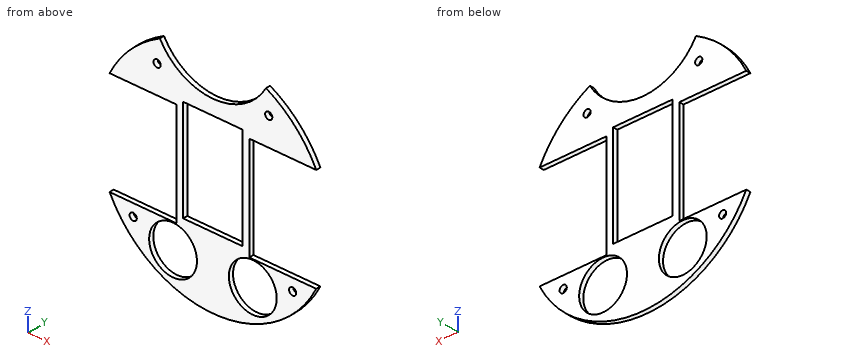
```python
from build123d import *

# Parameters (mm, degrees)
BOSS_EXTRUDE1_DEPTH  = 2.9
SOLENOID_PLACEMENT_W = 37.4
SOLENOID_PLACEMENT_H = 63.8
CUT_EXTRUDE1_DEPTH   = 103.571487266
CUT_EXTRUDE3_DEPTH   = 103.571487266
SKETCH7_R            = 15
CUT_EXTRUDE6_DEPTH   = 98.286484159
SKETCH8_R            = 2.25
CUT_EXTRUDE7_DEPTH   = 98.286484159


with BuildPart() as part:
    # Sketch1 → Boss-Extrude1 (new body)
    with BuildSketch(Plane(origin=(0, 0, 0), x_dir=(1, 0, 0), z_dir=(0, 1, 0))):
        with BuildLine():
            ThreePointArc((33.29110537, -64.404598464), (0, 72.5), (-33.29110537, -64.404598464))
            ThreePointArc((-33.29110537, -64.404598464), (0, -44.989799638), (33.29110537, -64.404598464))
        make_face()
    extrude(amount=BOSS_EXTRUDE1_DEPTH)

    # solenoid placement → Cut-Extrude1 (cut, through all)
    with BuildSketch(Plane(origin=(0, 2.9, 0), x_dir=(1, 0, 0), z_dir=(0, 1, 0))):
        with Locations((0, -3.8)):
            Rectangle(SOLENOID_PLACEMENT_W, SOLENOID_PLACEMENT_H)
    extrude(amount=-CUT_EXTRUDE1_DEPTH, mode=Mode.SUBTRACT)

    # Sketch3 → Cut-Extrude3 (cut, through all)
    with BuildSketch(Plane(origin=(0, 2.9, 0), x_dir=(1, 0, 0), z_dir=(0, 1, 0))):
        with BuildLine():
            Line((-34.63, -32.5), (-22.83, -32.5))
            Line((-22.83, -32.5), (-22.83, 32.5))
            Line((-22.83, 32.5), (-64.807406984, 32.5))
            ThreePointArc((-64.807406984, 32.5), (-72.5, 0), (-64.807406984, -32.5))
            Line((-64.807406984, -32.5), (-34.63, -32.5))
        make_face()
        with BuildLine():
            Line((22.83, -32.5), (22.83, 32.5))
            Line((22.83, 32.5), (64.807406984, 32.5))
            ThreePointArc((64.807406984, 32.5), (72.5, 0), (64.807406984, -32.5))
            Line((64.807406984, -32.5), (34.63, -32.5))
            Line((34.63, -32.5), (22.83, -32.5))
        make_face()
    extrude(amount=-CUT_EXTRUDE3_DEPTH, mode=Mode.SUBTRACT)

    # Sketch7 → Cut-Extrude6 (cut, through all)
    with BuildSketch(Plane(origin=(0, 2.9, 0), x_dir=(1, 0, 0), z_dir=(0, 1, 0))):
        with Locations(Location((25, 48, 0), (0, 0, 270))):
            Circle(SKETCH7_R)
        with Locations(Location((-25, 48, 0), (0, 0, 270))):
            Circle(SKETCH7_R)
    extrude(amount=-CUT_EXTRUDE6_DEPTH, mode=Mode.SUBTRACT)

    # Sketch8 → Cut-Extrude7 (cut, through all)
    with BuildSketch(Plane(origin=(0, 2.9, 0), x_dir=(1, 0, 0), z_dir=(0, 1, 0))):
        with Locations(Location((35, -50, 0), (0, 0, 270))):
            Circle(SKETCH8_R)
        with Locations(Location((-35, -50, 0), (0, 0, 270))):
            Circle(SKETCH8_R)
        with Locations(Location((-50, 40, 0), (0, 0, 270))):
            Circle(SKETCH8_R)
        with Locations(Location((50, 40, 0), (0, 0, 270))):
            Circle(SKETCH8_R)
    extrude(amount=-CUT_EXTRUDE7_DEPTH, mode=Mode.SUBTRACT)


solid = part.part
```
The model under review builds one solid part; all positions refer to its coordinate system, in mm. Round coordinates to 2 decimals unless told otherwise and drop trailing zeros. Loops run counter-clockwise (first coordinate to the right, second up) from the corner with the lowest first, then second, coordinate; pieces in that order, holes last. Notation, with made-up numbers: M 49.5,48.25 L 68.5,48.25 A29 ccw 68.5,73.25 Z; hole C -6.75,76 d3. An arc over 180 degrees is marked long. Write item = value, one per line.
Item 1: Insertion check: P1, Ø0.9, axis at x = -44, y = 1.5, coming from the +Z side; P2, Ø1.4, axis at x = 38.5, y = 1.5, coming from the -Z side; P3, Ø0.9, axis at x = 2, y = 2, coming from the -Z side. Each pin has a flat end and moves straight along its axis. Give the tip position at first contact, or say it passes through.
Return value:
P1 = 57.96
P2 = -61.87
P3 = -72.48
Item 2: Take a section at B-B on z = -23. Write out the cut boundary in (x, y).
Return value:
outline = M -22.83,0 L -18.7,0 L -18.7,2.9 L -22.83,2.9 Z; M 18.7,0 L 22.83,0 L 22.83,2.9 L 18.7,2.9 Z
Item 3: Take a section at D-D on z = 50. Write out the cut boundary in (x, y).
Return value:
outline = M -52.5,0 L -37.25,0 L -37.25,2.9 L -52.5,2.9 Z; M -32.75,0 L -18.93,0 L -18.93,2.9 L -32.75,2.9 Z; M 18.93,0 L 32.75,0 L 32.75,2.9 L 18.93,2.9 Z; M 37.25,0 L 52.5,0 L 52.5,2.9 L 37.25,2.9 Z
Item 4: For line 1 (Z direction, x = 1.5, y = 1.7); line 2 (X direction, y = 1.5, z = 50); line 3 (X direction, y = 0.8, z = -40), list the stretches that pass through material, from the lowest coordinate up. Write a range as [from, to].
Return value:
line_1 = [-72.48, -28.1], [35.7, 45.02]
line_2 = [-52.5, -37.25], [-32.75, -18.93], [18.93, 32.75], [37.25, 52.5]
line_3 = [-60.47, -52.25], [-47.75, -37.69], [-12.31, 12.31], [37.69, 47.75], [52.25, 60.47]
Item 5: Take a section at C-C on y = 1.7. Write out the cut boundary in (x, z).
Return value:
outline = M -64.81,-32.5 A72.5 ccw 64.81,-32.5 L 22.83,-32.5 L 22.83,32.5 L 64.81,32.5 A72.5 ccw 33.29,64.4 A38.25 cw -33.29,64.4 A72.5 ccw -64.81,32.5 L -22.83,32.5 L -22.83,-32.5 Z; hole C -50,-40 d4.5; hole C -25,-48 d30; hole C -35,50 d4.5; hole M -18.7,-28.1 L 18.7,-28.1 L 18.7,35.7 L -18.7,35.7 Z; hole C 25,-48 d30; hole C 35,50 d4.5; hole C 50,-40 d4.5
Item 6: Take a section at A-A on x = -50. Write out the cut boundary in (y, z).
Return value:
outline = M 0,-52.5 L 2.9,-52.5 L 2.9,-42.25 L 0,-42.25 Z; M 0,-37.75 L 2.9,-37.75 L 2.9,-32.5 L 0,-32.5 Z; M 0,32.5 L 2.9,32.5 L 2.9,52.5 L 0,52.5 Z
